Autodesk Inventor part; units mm, degrees
ref_plane "YZ Plane" through (0, 0, 0) normal (1, 0, 0) x (0, 1, 0)
ref_plane "XZ Plane" through (0, 0, 0) normal (0, 1, 0) x (-1, 0, 0)
ref_plane "XY Plane" through (0, 0, 0) normal (0, 0, 1) x (1, 0, 0)
sketch "Эскиз1" plane through (0, 0, 0) normal (0, 0, 1) x (1, 0, 0)
  line L0 (0, 0) -> (0, 72)
  line L1 (0, 72) -> (5, 72)
  line L2 (5, 72) -> (5, 62)
  line L3 (5, 62) -> (5.5, 62)
  line L4 (5.5, 62) -> (8, 17)
  line L5 (8, 17) -> (8, 12)
  line L6 (8, 12) -> (5, 12)
  line L7 (5, 12) -> (5, 0)
  line L8 (5, 0) -> (0, 0)
  line L9 (-5, 0) -> (-5, 12) construction
  line L10 (-5, 4) -> (6, 6.9474)
  line L11 (-5, 2.4471) -> (6, 5.3945)
  line L12 (-5, 4) -> (-5, 2.4471)
  line L13 (6, 6.9474) -> (6, 5.3945)
  dimension "d0" = 72
  dimension "d1" = 10
  dimension "d2" = 45
  dimension "d3" = 16
  dimension "d4" = 10
  dimension "d5" = 12
  dimension "d6" = 11
  dimension "d7" = 10
  dimension "d8" = 10
  dimension "d9" = 8
  dimension "d10" = 3
  dimension "d11" = 15
  dimension "d14" = 1
revolve "Вращение1" add sketch "Эскиз1" angle 360 about axis through (0, 0, 0) along (0, 1, 0) contours L0 L11 L7 L8 | L0 L10 L7 L11 | L0 L1 L2 L3 L4 L5 L6 L7 L10
revolve "Вращение2" cut sketch "Эскиз1" angle 360 about axis through (-5, 4, 0) along (0.9659258, 0.258819, 0) contours L11 L12 L10 L0 | L0 L10 L7 L11 | L7 L10 L13 L11
thread "Резьба1"
chamfer "Фаска1" distance 1.6 angle 45 1 edges at (-5, 72, 0)
chamfer "Фаска2" distance 1 angle 45 1 edges at (-5, 0, 0)
equation "\"d8\" = d4"
properties part number "Рукоятка"
The listing builds one solid part. Answer for the finished solid, in the listing's coordinates (mm). A direction names the side the tool comes from. Round coordinates to 2 decimals unless told otherwise and drop trailing zeros. Write each loop counter-clockwise with the first axis right and the second up, starting at its lowest first coordinate (ties: lowest second). Pieces come first, ordered by that corner, then holes. Notation, with made-up numbers: (-22.75, 45.5) - (12.25, 45.5) arc R10 ccw to (12.25, 64.5) - close; hole circle Ø6 at (11.5, 67). An arc over 180 degrees is marked (long way). Use one line per item in the form item = value. Start each with the question number.
Item 1: A cutting plane is placed at B-B (y = 30.5). Write down the section's boundary in (x, z).
Item 2: Flat-ended cylindrical pins translate along their axes: pin 1 Ø3 at (y, z) = (18, -5) entering from +X; pin 2 Ø4 at (x, z) = (-2.5, 6) entering from +Y; pin 3 Ø3 at (y, z) = (28, -2.5) entering from +X. Find the tip coordinate at first contact, or state that the pin passes through.
Item 3: Find the intervals of material crossed by line 1 (Y direction, x = 0.5, z = 1.25); line 2 (Y direction, x = 4.5, z = -2.5); line 3 (Y direction, x = -3.75, z = 0), in increasing order. Write a range as [from, to].
Item 4: Determine the mould class of faces 4 (the cylindrical face through (0.284, 4.581, -1.265)), 5 (the cylindrical face through (-1.73, 14.46, -7.81)), 6 (the flat face through (0, 0, 0)) for opening direction X: +X half, -X half, draft (parallel to the pull), parting line (faces both ways), or undercut.
Item 5: A cutting plane is placed at C-C (y = 66). Write down the section's boundary in (x, z), plus the area to 3 significant figures.
Item 6: A tool of negligible diameter and unlimited length cuts with its end or side. For faces 1 (the flat face through (0, 72, 0)), 2 (the cylindrical face through (4.619, 6.423, -1.915)), 3 (the flat face through (1.6, 62, 4.9)), from which of +Z, -Z, +X, -X, +Y, -Y can it reach the whole face along a straight path? Write none if from no direction.
Item 7: A cutting plane is placed at A-A (z = 0). Write down the section's boundary in (x, y).
The answers:
q1.outline = circle Ø14.5 at (0, 0)
q2.pin_1 = 7.14
q2.pin_2 = 70.9
q2.pin_3 = 7.34
q3.line_1 = [0, 4.62], [6.33, 72]
q3.line_2 = [12, 62]
q3.line_3 = [0, 2.78], [5.89, 71.65]
q4.face_4 = undercut
q4.face_5 = parting line
q4.face_6 = draft
q5.outline = circle Ø10 at (0, 0)
q5.area = 78.5 mm^2
q6.face_1 = +Z, -Z, +X, -X, +Y
q6.face_2 = -Y
q6.face_3 = +Y
q7.outline = (-8, 12) - (-5, 12) - (-5, 5.55) - (5, 8.23) - (5, 12) - (8, 12) - (8, 17) - (5.5, 62) - (5, 62) - (5, 70.4) - (3.4, 72) - (-3.4, 72) - (-5, 70.4) - (-5, 62) - (-5.5, 62) - (-8, 17) - close; (-5, 1) - (-4, 0) - (4, 0) - (5, 1) - (5, 5.13) - (-5, 2.45) - close
